```python
from build123d import *

# Parameters (mm, degrees)
F0_R     = 24.25
F1_DEPTH = 6


with BuildPart() as f1:
    # F0 (on Front) → F1 (new body)
    with BuildSketch(Plane.XZ):
        Circle(F0_R)
        with BuildLine():
            ThreePointArc((3, 9.539392), (8.062258, 5.91608), (10, 0))
            ThreePointArc((10, 0), (8.062258, -5.91608), (3, -9.539392))
            Line((3, -9.539392), (3, -12.5))
            Line((3, -12.5), (-3, -12.5))
            Line((-3, -12.5), (-3, -9.539392))
            ThreePointArc((-3, -9.539392), (-10, 0), (-3, 9.539392))
            Line((-3, 9.539392), (-3, 12.5))
            Line((-3, 12.5), (3, 12.5))
            Line((3, 12.5), (3, 9.539392))
        make_face(mode=Mode.SUBTRACT)
    extrude(amount=F1_DEPTH)


solid = f1.part
```
Could you check a few things on this model? Use its own coordinates, in mm. A direction names the side the tool comes from. Coordinates: 2 decimals unless noted, no trailing zeros. Loops run counter-clockwise (first coordinate to the right, second up) from the corner with the lowest first, then second, coordinate; pieces in that order, holes last.
1) Please list where these lines run through material, in increasing order: line 1 along X through (y, z) = (-2.3, 11); line 2 along X through (y, z) = (-5.25, 8).
Reported:
line 1: x = -21.61 to -3, 3 to 21.61
line 2: x = -22.89 to -6, 6 to 22.89
2) Imagine slicing it at A-A (x = 0). List the corners of the cut face in (y, z) for me, and give its area (3 significant figures).
Reported:
outline: (-6, -24.25) - (0, -24.25) - (0, -12.5) - (-6, -12.5) - close; (-6, 12.5) - (0, 12.5) - (0, 24.25) - (-6, 24.25) - close
area: 141 mm2
3) Which directions (+Z, -Z, +X, -X, +Y, -Y) give clear straight access to the entire face, cutting with the end or side of a thin tool? Please do faces 4 (the face through (10.4, -6, 0.3)), 5 (the face through (3, -3, -11)).
Reported:
face 4: +Z, -Z, +X, -X, -Y
face 5: +Y, -Y
4) Will these pins go through, and if not, where does the flat tip stop? pin 1 Ø2 at (y, z) = (-5.5, 2.5) entering from -X; pin 2 Ø2 at (y, z) = (-4.5, -10.5) entering from +X; pin 3 Ø3.5 at (y, z) = (-4, -11) entering from -X.
Reported:
pin 1: stops at x = -24.2
pin 2: stops at x = 22.31
pin 3: stops at x = -22.42
5) Imagine slicing it at D-D (x = -18). List the corners of the cut face in (y, z) for me, and give its area (3 significant figures).
Reported:
outline: (-6, -16.25) - (0, -16.25) - (0, 16.25) - (-6, 16.25) - close
area: 195 mm2
6) Imagine slicing it at B-B (z = -1). List the corners of the cut face in (x, y) for me.
Reported:
outline: (-24.23, -6) - (-9.95, -6) - (-9.95, 0) - (-24.23, 0) - close; (9.95, -6) - (24.23, -6) - (24.23, 0) - (9.95, 0) - close
7) Thinking about a two-plate mould opening in X: for faces 1 (the face through (-3, -3, -11)), 2 (the face through (10.4, 0, 0.3)), 3 (the face through (11.19, -2.958, -21.514)), which applies, released by +X, released by -X, zero draft, split by the parting line, or undercut?
Reported:
face 1: undercut
face 2: zero draft
face 3: split by the parting line
8) Imagine slicing it at C-C (y = -1.1). List the corners of the cut face in (x, z) for me, and give its area (3 significant figures).
Reported:
outline: circle Ø48.5 at (0, 0); hole (-3, -12.5) - (3, -12.5) - (3, -9.54) arc R10 ccw to (10, 0) arc R10 ccw to (3, 9.54) - (3, 12.5) - (-3, 12.5) - (-3, 9.54) arc R10 ccw to (-3, -9.54) - close
area: 1,500 mm2
